Geometry check sheet. Reference: the model listing, model coordinates, mm. Face numbers are marked on the shaded views. A direction names the side the tool comes from. Round coordinates to 2 decimals unless told otherwise and drop trailing zeros. Write each loop counter-clockwise with the first axis right and the second up, starting at its lowest first coordinate (ties: lowest second). Pieces come first, ordered by that corner, then holes. Notation, with made-up numbers: (8.25, 15.25) -> (20.25, 15.25) arc R18 cw to (20.25, 23.25) -> close; hole circle Ø4 at (78.5, 64.25). An arc over 180 degrees is marked (long way). One line per question, with ' | ' between items.
```python
from build123d import *

# Parameters (mm, degrees)
SKETCH1_W           = 250
SKETCH1_H           = 150
BOSS_EXTRUDE1_DEPTH = 2
SKETCH2_R           = 10
CUT_EXTRUDE1_DEPTH  = 2
CUT_EXTRUDE46_DEPTH = 10
CUT_EXTRUDE59_DEPTH = 10
SKETCH9_R           = 2.5
CUT_EXTRUDE60_DEPTH = 10
SKETCH19_R          = 1.5
CUT_EXTRUDE63_DEPTH = 10
SKETCH20_W          = 250
SKETCH20_H          = 150
SKETCH20_W_2        = 240
SKETCH20_H_2        = 140
BOSS_EXTRUDE5_DEPTH = 40


with BuildPart() as part:
    # Sketch1 → Boss-Extrude1 (new body)
    with BuildSketch(Plane(origin=(0, 0, 0), x_dir=(1, 0, 0), z_dir=(0, 1, 0))):
        Rectangle(SKETCH1_W, SKETCH1_H)
    extrude(amount=BOSS_EXTRUDE1_DEPTH)

    # Sketch2 → Cut-Extrude1 (cut)
    with BuildSketch(Plane(origin=(0, 2, 0), x_dir=(1, 0, 0), z_dir=(0, 1, 0))):
        with Locations(Location((0, 0, 0), (0, 0, 270))):
            Circle(SKETCH2_R)
    extrude(amount=-CUT_EXTRUDE1_DEPTH, mode=Mode.SUBTRACT)

    # Sketch7 → Cut-Extrude46 (cut)
    with BuildSketch(Plane(origin=(0, 2, 0), x_dir=(1, 0, 0), z_dir=(0, 1, 0))):
        with BuildLine():
            Line((102.5, 59), (102.5, 49))
            ThreePointArc((102.5, 49), (100, 46.5), (97.5, 49))
            Line((97.5, 49), (97.5, 59))
            ThreePointArc((97.5, 59), (100, 61.5), (102.5, 59))
        make_face()
        with BuildLine():
            Line((77.5, 59), (77.5, 49))
            ThreePointArc((77.5, 49), (80, 46.5), (82.5, 49))
            Line((82.5, 49), (82.5, 59))
            ThreePointArc((82.5, 59), (80, 61.5), (77.5, 59))
        make_face()
        with BuildLine():
            Line((82.5, -1), (82.5, 9))
            ThreePointArc((82.5, 9), (80, 11.5), (77.5, 9))
            Line((77.5, 9), (77.5, -1))
            ThreePointArc((77.5, -1), (80, -3.5), (82.5, -1))
        make_face()
        with BuildLine():
            Line((97.5, -1), (97.5, 9))
            ThreePointArc((97.5, 9), (100, 11.5), (102.5, 9))
            Line((102.5, 9), (102.5, -1))
            ThreePointArc((102.5, -1), (100, -3.5), (97.5, -1))
        make_face()
    extrude(amount=-CUT_EXTRUDE46_DEPTH, mode=Mode.SUBTRACT)

    # Sketch3 → Cut-Extrude59 (cut)
    with BuildSketch(Plane.XZ):
        with BuildLine():
            Line((-40, -9), (-40, 1))
            ThreePointArc((-40, 1), (-42.5, 3.5), (-45, 1))
            Line((-45, 1), (-45, -9))
            ThreePointArc((-45, -9), (-42.5, -11.5), (-40, -9))
        make_face()
        with BuildLine():
            Line((-40, -49), (-40, -59))
            ThreePointArc((-40, -59), (-42.5, -61.5), (-45, -59))
            Line((-45, -59), (-45, -49))
            ThreePointArc((-45, -49), (-42.5, -46.5), (-40, -49))
        make_face()
        with BuildLine():
            Line((40, -9), (40, 1))
            ThreePointArc((40, 1), (42.5, 3.5), (45, 1))
            Line((45, 1), (45, -9))
            ThreePointArc((45, -9), (42.5, -11.5), (40, -9))
        make_face()
        with BuildLine():
            Line((40, -49), (40, -59))
            ThreePointArc((40, -59), (42.5, -61.5), (45, -59))
            Line((45, -59), (45, -49))
            ThreePointArc((45, -49), (42.5, -46.5), (40, -49))
        make_face()
    extrude(amount=-CUT_EXTRUDE59_DEPTH, mode=Mode.SUBTRACT)

    # Sketch9 → Cut-Extrude60 (cut)
    with BuildSketch(Plane(origin=(0, 2, 0), x_dir=(1, 0, 0), z_dir=(0, 1, 0))):
        with Locations(Location((-30, 15, 0), (0, 0, 270))):
            Circle(SKETCH9_R)
        with Locations(Location((-30, -15, 0), (0, 0, 270))):
            Circle(SKETCH9_R)
        with Locations(Location((30, -15, 0), (0, 0, 90))):
            Circle(SKETCH9_R)
        with Locations(Location((30, 15, 0), (0, 0, 90))):
            Circle(SKETCH9_R)
    extrude(amount=-CUT_EXTRUDE60_DEPTH, mode=Mode.SUBTRACT)

    # Sketch19 → Cut-Extrude63 (cut)
    with BuildSketch(Plane(origin=(0, 2, 0), x_dir=(1, 0, 0), z_dir=(0, 1, 0))):
        with Locations(Location((105, -55, 0), (0, 0, 270))):
            Circle(SKETCH19_R)
        with Locations(Location((95, -55, 0), (0, 0, 270))):
            Circle(SKETCH19_R)
        with Locations(Location((-95, -55, 0), (0, 0, 90))):
            Circle(SKETCH19_R)
        with Locations(Location((-105, -55, 0), (0, 0, 90))):
            Circle(SKETCH19_R)
    extrude(amount=-CUT_EXTRUDE63_DEPTH, mode=Mode.SUBTRACT)

    # Sketch20 → Boss-Extrude5 (add)
    with BuildSketch(Plane.XZ):
        Rectangle(SKETCH20_W, SKETCH20_H)
        Rectangle(SKETCH20_W_2, SKETCH20_H_2, mode=Mode.SUBTRACT)
    extrude(amount=BOSS_EXTRUDE5_DEPTH)


solid = part.part
```
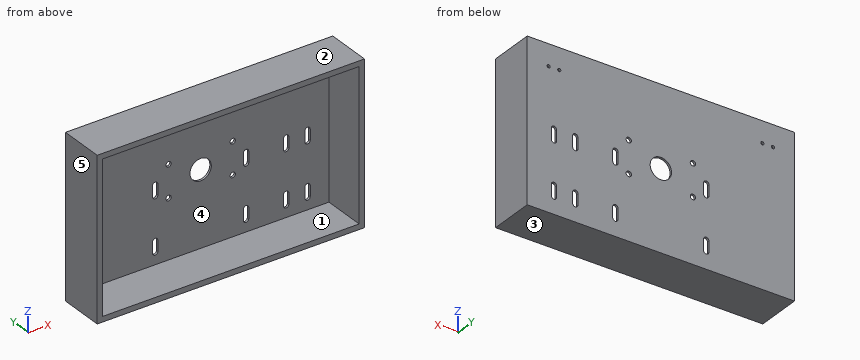
(1) Sectioned sample at A-A on x = -30. Record the cut outline in (y, z), then the cut area to 3 significant figures.
Resolved:
outline: (-40, -75) -> (2, -75) -> (2, -17.5) -> (0, -17.5) -> (0, -70) -> (-40, -70) -> close; (-40, 70) -> (0, 70) -> (0, 17.5) -> (2, 17.5) -> (2, 75) -> (-40, 75) -> close; (0, -12.5) -> (2, -12.5) -> (2, 12.5) -> (0, 12.5) -> close | area: 680 mm2
(2) Sectioned sample at C-C on y = -7. Record the cut outline in (x, z).
Resolved:
outline: (-125, -75) -> (125, -75) -> (125, 75) -> (-125, 75) -> close; hole (-120, -70) -> (120, -70) -> (120, 70) -> (-120, 70) -> close
(3) Access from +Z, -Z, +X, -X, +Y, -Y to the whole of each face (thin tool, end or side, straight path). Record for the marked faces 1 and 2.
Resolved:
face 1: -Y | face 2: +Z, +X, -X, +Y, -Y
(4) Sectioned sample at B-B on z = -15. Record the cut outline in (x, y), then the cut area to 3 significant figures.
Resolved:
outline: (-125, -40) -> (-120, -40) -> (-120, 0) -> (-32.5, 0) -> (-32.5, 2) -> (-125, 2) -> close; (-27.5, 0) -> (27.5, 0) -> (27.5, 2) -> (-27.5, 2) -> close; (32.5, 0) -> (120, 0) -> (120, -40) -> (125, -40) -> (125, 2) -> (32.5, 2) -> close | area: 880 mm2
(5) Material ranges on line 1 (X direction, y = 0.95, z = 15); line 2 (X direction, y = 0.65, z = 55); line 3 (Z direction, x = 30, y = 1.6), recorded low to high.
Resolved:
line 1: x = -125 to -32.5, -27.5 to 27.5, 32.5 to 125 | line 2: x = -125 to -106.5, -103.5 to -96.5, -93.5 to 93.5, 96.5 to 103.5, 106.5 to 125 | line 3: z = -75 to -17.5, -12.5 to 12.5, 17.5 to 75
(6) Sectioned sample at D-D on z = 41. Record the cut outline in (x, y).
Resolved:
outline: (-125, -40) -> (-120, -40) -> (-120, 0) -> (120, 0) -> (120, -40) -> (125, -40) -> (125, 2) -> (-125, 2) -> close
(7) Draft check along Z on the marked faces 3, 4 and 5. Enter one of: +Z half, -Z half, draft (parallel to the pull), parting line (faces both ways), or undercut.
Resolved:
face 3: -Z half | face 4: undercut | face 5: draft
(8) Go/stop test with a flat-tipped pin: pin 1 (5 mm diameter, centred on x = 105, z = 55, fed in from +Y). Record where the tip stops, or that it passes through.
Resolved:
pin 1: stops at y = 2
